```python
from build123d import *

# Parameters (mm, degrees)
SKETCH1_R           = 77.5
BOSS_EXTRUDE1_DEPTH = 6
SKETCH2_R           = 12.5
CUT_EXTRUDE1_DEPTH  = 110.765659475
SKETCH3_R           = 3.099503232
CUT_EXTRUDE2_DEPTH  = 5.228379
CIRPATTERN1_START   = 0.771620962
CIRPATTERN1_DEPTH   = 5.228379038


# Read off the part's stored shape, not the designer's step: CirPattern1
with BuildPart() as part:
    # Sketch1 → Boss-Extrude1 (new body)
    with BuildSketch(Plane(origin=(0, 0, 0), x_dir=(1, 0, 0), z_dir=(0, 1, 0))):
        with Locations(Location((0, 0, 0), (0, 0, 270))):
            Circle(SKETCH1_R)
    extrude(amount=BOSS_EXTRUDE1_DEPTH)

    # Sketch2 → Cut-Extrude1 (cut, through all)
    with BuildSketch(Plane(origin=(0, 0, 0), x_dir=(1, 0, 0), z_dir=(0, 1, 0))):
        with Locations(Location((0, 0, 0), (0, 0, 270))):
            Circle(SKETCH2_R)
    extrude(amount=CUT_EXTRUDE1_DEPTH, mode=Mode.SUBTRACT)

    # Sketch3 → Cut-Extrude2 (cut)
    with BuildSketch(Plane(origin=(0, 6, 0), x_dir=(1, 0, 0), z_dir=(0, 1, 0))):
        with Locations((-12.391135016, 0)):
            Circle(SKETCH3_R)
    extrude(amount=-CUT_EXTRUDE2_DEPTH, mode=Mode.SUBTRACT)

    # CirPattern1 outline → CirPattern1 (cut)
    with BuildSketch(Plane(origin=(0, 0, 0), x_dir=(1, 0, 0), z_dir=(0, 1, 0)).offset(CIRPATTERN1_START)):
        with BuildLine():
            ThreePointArc((-6.382234283, -10.747887493), (-8.838834765, -8.838834765), (-10.747887493, -6.382234283))
            ThreePointArc((-10.747887493, -6.382234283), (-10.95353535, -10.95353535), (-6.382234283, -10.747887493))
        make_face()
        with BuildLine():
            ThreePointArc((-6.382234283, 10.747887493), (-10.95353535, 10.95353535), (-10.747887493, 6.382234283))
            ThreePointArc((-10.747887493, 6.382234283), (-8.838834765, 8.838834765), (-6.382234283, 10.747887493))
        make_face()
        with BuildLine():
            ThreePointArc((3.086982989, -12.11282527), (0, -12.5), (-3.086982989, -12.11282527))
            ThreePointArc((-3.086982989, -12.11282527), (0, -15.490638248), (3.086982989, -12.11282527))
        make_face()
        with BuildLine():
            ThreePointArc((3.086982989, 12.11282527), (0, 15.490638248), (-3.086982989, 12.11282527))
            ThreePointArc((-3.086982989, 12.11282527), (0, 12.5), (3.086982989, 12.11282527))
        make_face()
        with BuildLine():
            ThreePointArc((10.747887493, -6.382234283), (8.838834765, -8.838834765), (6.382234283, -10.747887493))
            ThreePointArc((6.382234283, -10.747887493), (10.95353535, -10.95353535), (10.747887493, -6.382234283))
        make_face()
        with BuildLine():
            ThreePointArc((10.747887493, 6.382234283), (10.95353535, 10.95353535), (6.382234283, 10.747887493))
            ThreePointArc((6.382234283, 10.747887493), (8.838834765, 8.838834765), (10.747887493, 6.382234283))
        make_face()
        with BuildLine():
            ThreePointArc((12.11282527, 3.086982989), (12.5, 0), (12.11282527, -3.086982989))
            ThreePointArc((12.11282527, -3.086982989), (15.490638248, 0), (12.11282527, 3.086982989))
        make_face()
    extrude(amount=CIRPATTERN1_DEPTH, mode=Mode.SUBTRACT)


solid = part.part
```
Can you work these out from the model? Positions are in its coordinate system, mm. A direction names the side the tool comes from. Coordinates: 2 decimals unless noted, no trailing zeros. Loops run counter-clockwise (first coordinate to the right, second up) from the corner with the lowest first, then second, coordinate; pieces in that order, holes last.
Item 1: Suppose I cut it at C-C (y = 2.8). Please give me the cut outline in (x, z).
Answers below:
outline: circle Ø155 at (0, 0); hole (-12.11, -3.09) arc R12.5 ccw to (-10.75, -6.38) arc R3.1 ccw (long way) to (-6.38, -10.75) arc R12.5 ccw to (-3.09, -12.11) arc R3.1 ccw (long way) to (3.09, -12.11) arc R12.5 ccw to (6.38, -10.75) arc R3.1 ccw (long way) to (10.75, -6.38) arc R12.5 ccw to (12.11, -3.09) arc R3.1 ccw (long way) to (12.11, 3.09) arc R12.5 ccw to (10.75, 6.38) arc R3.1 ccw (long way) to (6.38, 10.75) arc R12.5 ccw to (3.09, 12.11) arc R3.1 ccw (long way) to (-3.09, 12.11) arc R12.5 ccw to (-6.38, 10.75) arc R3.1 ccw (long way) to (-10.75, 6.38) arc R12.5 ccw to (-12.11, 3.09) arc R3.1 ccw (long way) to start
Item 2: Please list where these lines run through material, in increasing order: L1, parallel to X at y = 2.45, z = 0; L2, parallel to X at y = 3.1, z = 3.5; L3, parallel to Z at x = -2, y = 3.2.
Answers below:
L1: x = -77.5 to -15.49, 15.49 to 77.5
L2: x = -77.42 to -12, 12 to 77.42
L3: z = -77.47 to -14.76, 14.76 to 77.47
Item 3: Which directions (+Z, -Z, +X, -X, +Y, -Y) give clear straight access to the entire face, cutting with the end or side of a thin tool? Please do faces 4 (the face through (-4.788, 2.291, 11.547)), 5 (the face through (-14, 0.772, 0)).
Answers below:
face 4: +Y, -Y
face 5: +Y
Item 4: Suppose I cut it at D-D (x = 38). Please give me the cut outline in (y, z).
Answers below:
outline: (0, -67.54) - (6, -67.54) - (6, 67.54) - (0, 67.54) - close
Item 5: I'm going to push flat-ended pins straight in: pin 1 (1 mm diameter, centred on x = 0.5, z = 14, fed in from +Y); pin 2 (1.5 mm diameter, centred on y = 3.5, z = 38.5, fed in from -X). Where does each tip first touch, or does it pass through?
Answers below:
pin 1: stops at y = 0.77
pin 2: stops at x = -67.68
Item 6: Suppose I cut it at A-A (z = 0). Please give me the cut outline in (x, y), then the cut area to 3 significant figures.
Answers below:
outline: (-77.5, 0) - (-12.5, 0) - (-12.5, 0.77) - (-15.49, 0.77) - (-15.49, 6) - (-77.5, 6) - close; (12.5, 0) - (77.5, 0) - (77.5, 6) - (15.49, 6) - (15.49, 0.77) - (12.5, 0.77) - close
area: 749 mm2
Item 7: Suppose I cut it at B-B (x = 0). Please give me the cut outline in (y, z).
Answers below:
outline: (0, -77.5) - (6, -77.5) - (6, -15.49) - (0.77, -15.49) - (0.77, -12.5) - (0, -12.5) - close; (0, 12.5) - (0.77, 12.5) - (0.77, 15.49) - (6, 15.49) - (6, 77.5) - (0, 77.5) - close
Item 8: If we mould it in two halves opening along Z, with no side actions, what happens to faces 1 (the face through (-29.68, 2.96, 71.59)), 2 (the face through (0, 0.772, 14)), 3 (the face through (-16, 6, -1))? For each: released by +Z, released by -Z, zero draft, split by the parting line, or undercut.
Answers below:
face 1: split by the parting line
face 2: undercut
face 3: zero draft
